```python
from build123d import *

# Parameters (mm, degrees)
SKETCH_1_W          = 50
SKETCH_1_H          = 60
EXTRUDE_1_DEPTH     = 16
SKETCH_2_R          = 3.25
CUT_EXTRUDE_1_DEPTH = 100
SKETCH_3_R          = 1.5
CUT_EXTRUDE_2_DEPTH = 100
EXTRUDE_2_DEPTH     = 60
SKETCH_5_R          = 1.5
CUT_EXTRUDE_3_DEPTH = 60


with BuildPart() as part:
    # 草圖1 → 填料-伸長1 (new body)
    with BuildSketch(Plane(origin=(0, 0, 0), x_dir=(1, 0, 0), z_dir=(0, 1, 0))):
        with Locations((25, 30)):
            Rectangle(SKETCH_1_W, SKETCH_1_H)
    extrude(amount=EXTRUDE_1_DEPTH)

    # 草圖2 → 除料-伸長1 (cut)
    with BuildSketch(Plane(origin=(0, 0, -60), x_dir=(-1, 0, 0), z_dir=(0, 0, -1))):
        with Locations((-45, 8)):
            Circle(SKETCH_2_R)
        with Locations((-5, 8)):
            Circle(SKETCH_2_R)
    extrude(amount=-CUT_EXTRUDE_1_DEPTH, mode=Mode.SUBTRACT)

    # 草圖3 → 除料-伸長2 (cut)
    with BuildSketch(Plane(origin=(0, 16, 0), x_dir=(1, 0, 0), z_dir=(0, 1, 0))):
        with Locations(Location((13, 10, 0), (0, 0, 270))):
            Circle(SKETCH_3_R)
        with Locations(Location((13, 50, 0), (0, 0, 270))):
            Circle(SKETCH_3_R)
    extrude(amount=-CUT_EXTRUDE_2_DEPTH, mode=Mode.SUBTRACT)

    # 草圖4 → 填料-伸長2 (add)
    with BuildSketch(Plane.XY):
        Polygon((0, 0), (-3, 3), (-3, 13), (0, 16), align=None)
        Polygon((53, 13), (50, 16), (50, 0), (53, 3), align=None)
    extrude(amount=-EXTRUDE_2_DEPTH)

    # 草圖5 → 除料-伸長3 (cut)
    with BuildSketch(Plane(origin=(0, 16, 0), x_dir=(1, 0, 0), z_dir=(0, 1, 0))):
        with Locations(Location((25, 20, 0), (0, 0, 270))):
            Circle(SKETCH_5_R)
        with Locations(Location((25, 40, 0), (0, 0, 270))):
            Circle(SKETCH_5_R)
    extrude(amount=-CUT_EXTRUDE_3_DEPTH, mode=Mode.SUBTRACT)


solid = part.part
```
Design review of the part built by this model. Coordinates are the model's own, in mm. Give positions to 0.01 mm unless a question says otherwise; leave off trailing zeros. Order: outer loops, then holes, each group sorted by start corner. A loop starts at its lowest first (then second) coordinate and runs counter-clockwise, first axis right, second up. Notation, with made-up numbers: M 80.5,-17.5 L 118.5,-17.5 A27 cw 118.5,12.5 Z; hole C 44.25,83 d7. An arc over 180 degrees is marked long. One line per question, with ' | ' between items. Start each with the question number.
Q1. We need section C-C (y = 9). Write out the cut boundary in (x, z).
Q2. We need section A-A (z = -10). Write out the cut boundary in (x, y).
Q3. We need section B-B (x = 5). Write out the cut boundary in (y, z), plus the area to 3 significant figures.
Q4. For L1, parallel to X at y = 8.25, z = -31.5; L2, parallel to X at y = 8.25, z = -50; L3, parallel to X at y = 10.5, z = -10, list the stretches that pass through material, from the lowest coordinate up. Write a range as [from, to].
Q5. For pin 1 Ø1.8 at (x, z) = (13, -10) entering from +Y, flat-tipped, find the tip position at first contact; note if it passes through.
Q6. The part is to be moulded in two halves that separate along Y. For faces 1 (the face through (25, 0, -30)), 2 (the face through (13.07, 8.11, -51.5)), 3 (the face through (41.9, 8.98, -30.42)), say which applies: +Y half, -Y half, draft (parallel to the pull), parting line (faces both ways), or undercut.
Q7. We need section D-D (x = 25). Write out the cut boundary in (y, z).
Returned:
1) outline: M -3,-60 L 1.91,-60 L 1.91,0 L -3,0 Z; M 8.09,-60 L 41.91,-60 L 41.91,0 L 8.09,0 Z; M 48.09,-60 L 53,-60 L 53,0 L 48.09,0 Z; hole C 13,-50 d3; hole C 13,-10 d3; hole C 25,-40 d3; hole C 25,-20 d3
2) outline: M -3,3 L 0,0 L 11.5,0 L 11.5,16 L 0,16 L -3,13 Z; M 14.5,0 L 50,0 L 53,3 L 53,13 L 50,16 L 14.5,16 Z; hole C 5,8 d6.5; hole C 45,8 d6.5
3) outline: M 0,-60 L 4.75,-60 L 4.75,0 L 0,0 Z; M 11.25,-60 L 16,-60 L 16,0 L 11.25,0 Z | area: 570 mm2
4) L1: [-3, 1.76], [8.24, 41.76], [48.24, 53] | L2: [-3, 1.76], [8.24, 11.5], [14.5, 41.76], [48.24, 53] | L3: [-3, 2.92], [7.08, 11.5], [14.5, 42.92], [47.08, 53]
5) pin 1: through
6) face 1: -Y half | face 2: draft | face 3: undercut
7) outline: M 0,-60 L 16,-60 L 16,-41.5 L 0,-41.5 Z; M 0,-38.5 L 16,-38.5 L 16,-21.5 L 0,-21.5 Z; M 0,-18.5 L 16,-18.5 L 16,0 L 0,0 Z
